The drawing under review shows one solid part. Ordinate dimensions are in mm from its lowest x, y, z. A direction names the side the tool comes from. Give positions to 0.01 mm unless a question says otherwise; leave off trailing zeros. Order: outer loops, then holes, each group sorted by start corner. A loop starts at its lowest first (then second) coordinate and runs counter-clockwise, first axis right, second up. Notation, with made-up numbers: (67.5, 32.25) - (100.5, 32.25) arc R17 ccw to (100.5, 39.25) - close; hole circle Ø9 at (65.5, 44). An arc over 180 degrees is marked (long way). Answer as a JSON object with one key per item and string values. Group by question number.
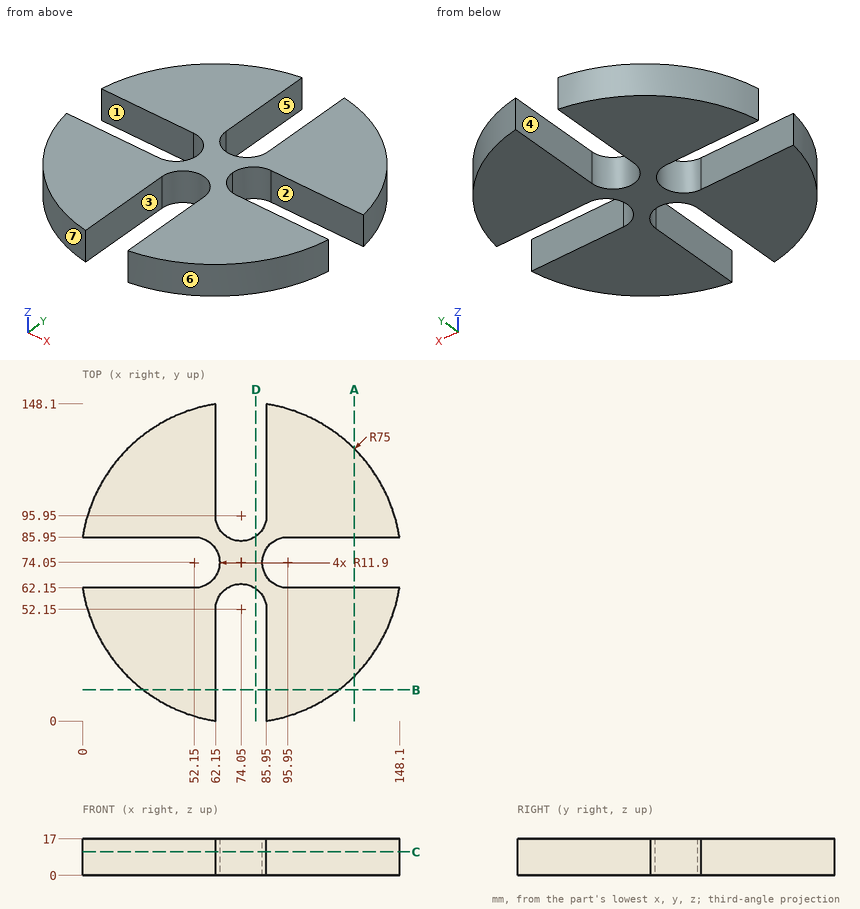
1) Consider section D-D (x = 81). Give the boundary of the cut face in (y, z), plus the area to 3 significant figures.
2) Consider section C-C (z = 11). Give the boundary of the cut face in (x, y), plus the area to 3 significant figures.
3) For line 1 (Y direction, x = 27, z = 15.75); line 2 (X direction, y = 28, z = 1); line 3 (Y direction, x = 62, z = 14.25) (1 decimal), list the stretches that pass through material, from the lowest coordinate up.
4) For the marked faces 1, 2, 3 and 4, list the 3-axis set-ups (+Z, -Z, +X, -X, +Y, -Y) from which the entire face can be reached by the end or side of a thin tool; tool diameter is ignored.
5) Mouldability with a two-part tool opening along X and no side actions: class the marked faces 5, 6 and 7 as released by +X, released by -X, zero draft, split by the parting line, or undercut.
6) Consider section A-A (x = 127). Give the boundary of the cut face in (y, z), plus the area to 3 significant figures.
7) For pin 1 (8.5 mm diameter, centred on y = 135, z = 7.5, fed in from +X); pin 2 (3 mm diameter, centred on x = 79.5, z = 8, fed in from -Y); pin 3 (8 mm diameter, centred on x = 30.5, z = 5, fed in from -Y) (1 decimal), all flat-tipped, find the tip position at first contact; note any pin that passes through.
8) Consider section B-B (y = 14.5). Give the boundary of the cut face in (x, z).
Result set:
{
 "1": {"outline": "(61.81, 0) - (86.29, 0) - (86.29, 17) - (61.81, 17) - close", "area": "416 mm2"},
 "2": {"outline": "(0, 62.15) arc R75 ccw to (62.15, 0) - (62.15, 52.15) arc R11.9 cw to (85.95, 52.15) - (85.95, 0) arc R75 ccw to (148.1, 62.15) - (95.95, 62.15) arc R11.9 cw to (95.95, 85.95) - (148.1, 85.95) arc R75 ccw to (85.95, 148.1) - (85.95, 95.95) arc R11.9 cw to (62.15, 95.95) - (62.15, 148.1) arc R75 ccw to (0, 85.95) - (52.15, 85.95) arc R11.9 cw to (52.15, 62.15) - close", "area": "11,800 mm2"},
 "3": {"line 1": "y = 15.64 to 62.15, 85.95 to 132.46", "line 2": "x = 14.85 to 62.15, 85.95 to 133.25", "line 3": "y = 0 to 67.4, 80.7 to 148.1"},
 "4": {"face 1": "+Z, -Z, -X", "face 2": "+Z, -Z, +X", "face 3": "+Z, -Z, -Y", "face 4": "+Z, -Z, +Y"},
 "5": {"face 5": "undercut", "face 6": "released by +X", "face 7": "released by -X"},
 "6": {"outline": "(20.93, 0) - (62.15, 0) - (62.15, 17) - (20.93, 17) - close; (85.95, 0) - (127.17, 0) - (127.17, 17) - (85.95, 17) - close", "area": "1,400 mm2"},
 "7": {"pin 1": "stops at x = 123.14", "pin 2": "stops at y = 61.81", "pin 3": "stops at y = 10.3"},
 "8": {"outline": "(28.46, 0) - (62.15, 0) - (62.15, 17) - (28.46, 17) - close; (85.95, 0) - (119.64, 0) - (119.64, 17) - (85.95, 17) - close"}
}
